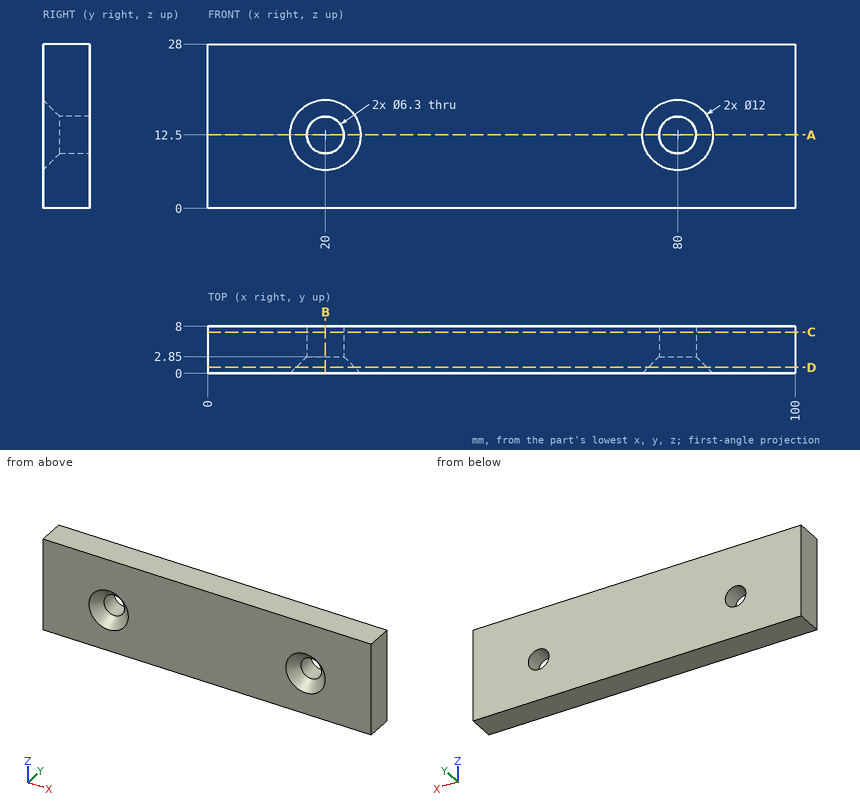
Check sheet for the drawn part. Datum: minimum x, y, z corner. Units: mm. Give positions to 0.01 mm unless a question says otherwise; leave off trailing zeros. Order: outer loops, then holes, each group sorted by start corner. A loop starts at its lowest first (then second) coordinate and runs counter-clockwise, first axis right, second up. Notation, with made-up numbers: (-15, 50) -> (38, 50) arc R26 cw to (38, 69) -> close; hole circle Ø10 at (58.5, -15). An arc over 180 degrees is marked (long way). Use a Markdown table: item, result.
1) Depth check by flat-ended pin: pin 1 Ø4 at (x, z) = (68, 12) entering from -Y; pin 2 Ø7 at (x, z) = (20, 12.5) entering from -Y. Enter the tip coordinate at first touch or a pass-through.
Results:
| item | result |
|---|---|
| pin 1 | y = 0 |
| pin 2 | y = 2.5 |
2) Section check A-A, the plane z = 12.5. Record the boundary of the cut face in (x, y), then the cut area to 3 significant figures.
Results:
| item | result |
|---|---|
| outline | (0, 0) -> (14, 0) -> (16.85, 2.85) -> (16.85, 8) -> (0, 8) -> close; (23.15, 2.85) -> (26, 0) -> (74, 0) -> (76.85, 2.85) -> (76.85, 8) -> (23.15, 8) -> close; (83.15, 2.85) -> (86, 0) -> (100, 0) -> (100, 8) -> (83.15, 8) -> close |
| area | 683 mm² |
3) Section check D-D, the plane y = 1. Record the boundary of the cut face in (x, z).
Results:
| item | result |
|---|---|
| outline | (0, 0) -> (100, 0) -> (100, 28) -> (0, 28) -> close; hole circle Ø10 at (20, 12.5); hole circle Ø10 at (80, 12.5) |
4) Section check C-C, the plane y = 7. Record the boundary of the cut face in (x, z), then the cut area to 3 significant figures.
Results:
| item | result |
|---|---|
| outline | (0, 0) -> (100, 0) -> (100, 28) -> (0, 28) -> close; hole circle Ø6.3 at (20, 12.5); hole circle Ø6.3 at (80, 12.5) |
| area | 2,740 mm² |
5) Section check B-B, the plane x = 20. Record the boundary of the cut face in (y, z).
Results:
| item | result |
|---|---|
| outline | (0, 0) -> (8, 0) -> (8, 9.35) -> (2.85, 9.35) -> (0, 6.5) -> close; (0, 18.5) -> (2.85, 15.65) -> (8, 15.65) -> (8, 28) -> (0, 28) -> close |
6) Material ranges on probe 1 along X at (y, z) = (4.35, 12.5); probe 2 along Z at (x, y) = (80, 6); probe 3 along X at (y, z) = (5.75, 11.5), recorded low to high.
Results:
| item | result |
|---|---|
| probe 1 | 0 to 16.85, 23.15 to 76.85, 83.15 to 100 |
| probe 2 | 0 to 9.35, 15.65 to 28 |
| probe 3 | 0 to 17.01, 22.99 to 77.01, 82.99 to 100 |
